Can you work these out from the model? Positions are in its coordinate system, mm. A direction names the side the tool comes from. Coordinates: 2 decimals unless noted, no trailing zeros. Write each loop counter-clockwise with the first axis right and the second up, starting at its lowest first coordinate (ties: lowest second). Pieces come first, ordered by that corner, then holes. Notation, with made-up numbers: (-18.75, 38) - (29.25, 38) arc R15 cw to (29.25, 51) - close; hole circle Ø10 at (72.5, 70). An arc over 180 degrees is marked (long way). Use one line per item in the form item = value. Start each with the question number.
(1) If we section it at D-D on y = -5: Please give me the cut outline in (x, z).
(2) On a 3-axis mill with a long thin cutter (end or side, diameter ignored), from which of +Z, -Z, +X, -X, +Y, -Y can I reach the whole of each face in a straight line? I mean faces 5 (the face through (51, 8, 1)), 6 (the face through (0.86, 15.1, 0.76)), 7 (the face through (41, -2, 2)), 8 (the face through (0.86, 0.9, 0.76)), 9 (the face through (10, -2, 2)). Say none if no direction works.
(3) If we section it at C-C on z = 2: Please give me the cut outline in (x, y).
(4) For pin 1 Ø0.8 at (x, z) = (15.5, 0.5) entering from +Y; pin 2 Ø0.8 at (x, z) = (46, 2.5) entering from -Y; pin 3 Ø1.5 at (y, z) = (-2.5, 0.5) entering from -X; pin 4 Ø1.2 at (y, z) = (-4, 2.5) entering from -X, each with a flat end and sliding along its axis, tell me the tip position at first contact or that it passes through.
(5) If I drill on probe 1 along X at (y, z) = (18, 2.25); probe 2 along X at (y, z) = (-5, 1.85); probe 3 along Y at (x, z) = (25.5, 1.9), over which ranges is the centre line in solid material (lowest first)? Write a range as from..to.
(6) If we section it at A-A on x = 25.5: Please give me the cut outline in (y, z).
(7) Thinking about a two-plate mould opening in Y: for faces 1 (the face through (-0.283, 17.024, 1.993)), 2 (the face through (23.6, 16.3, 1.5)), 3 (the face through (26, 20, 2)), 4 (the face through (51.04, 17.11, 1.99)), which applies, pulls with the +Y half, pulls with the -Y half, needs draft (parallel to the pull), parting line crosses it, or undercut?
(8) If we section it at B-B on y = 18: Please give me the cut outline in (x, z).
```python
from build123d import *

# Parameters (mm, degrees)
SKETCH_1_W                  = 51
SKETCH_1_H                  = 16
EXTRUDE_1_DEPTH             = 1.5
EXTRUDE_2_DEPTH             = 1.5
FILLET_2_R                  = 3
HOLE_WIZARD_M21_D           = 2
HOLE_WIZARD_M21_CSINK_D     = 3
HOLE_WIZARD_M21_CSINK_ANGLE = 90


with BuildPart() as part:
    # Эскиз1 → Бобышка-Вытянуть1 (new body)
    with BuildSketch(Plane.XY):
        with Locations((25.5, 8)):
            Rectangle(SKETCH_1_W, SKETCH_1_H)
    extrude(amount=EXTRUDE_1_DEPTH)

    # Эскиз2 → Бобышка-Вытянуть2 (add)
    with BuildSketch(Plane.XY.offset(1.5)):
        Polygon((3.5, 20), (47.5, 20), (53.5, 20), (53.5, 19.5), (53.5, -2), (28.75, -2), (28.75, -9), (21.75, -9), (21.75, -2), (-2.5, -2), (-2.5, 19.5), (-2.5, 20), align=None)
    extrude(amount=EXTRUDE_2_DEPTH)

    # Скругление2
    fillet_2_edges = [part.edges().sort_by_distance(p)[0] for p in [
        (0, 0, 0.75),
        (0, 16, 0.75),
        (51, 16, 0.75),
        (51, 0, 0.75),
    ]]
    fillet(fillet_2_edges, radius=FILLET_2_R)

    # Зенковка для  винта с полупотайной головкой M21 (through all)
    with Locations(Plane.XY.offset(3)):
        with Locations((25.5, -5), (-0.5, 18), (51.5, 18)):
            CounterSinkHole(HOLE_WIZARD_M21_D / 2, HOLE_WIZARD_M21_CSINK_D / 2, counter_sink_angle=HOLE_WIZARD_M21_CSINK_ANGLE)


solid = part.part
```
Reported:
q1.outline = (21.75, 1.5) - (24.5, 1.5) - (24.5, 2.5) - (24, 3) - (21.75, 3) - close; (26.5, 1.5) - (28.75, 1.5) - (28.75, 3) - (27, 3) - (26.5, 2.5) - close
q2.face_5 = -Z, +X, +Y, -Y
q2.face_6 = -Z, -X, +Y
q2.face_7 = +Z, -Z, +X, -Y
q2.face_8 = -Z, -X, -Y
q2.face_9 = +Z, -Z, -X, -Y
q3.outline = (-2.5, -2) - (21.75, -2) - (21.75, -9) - (28.75, -9) - (28.75, -2) - (53.5, -2) - (53.5, 20) - (-2.5, 20) - close; hole circle Ø2 at (-0.5, 18); hole circle Ø2 at (25.5, -5); hole circle Ø2 at (51.5, 18)
q4.pin_1 = 16
q4.pin_2 = -2
q4.pin_3 = through
q4.pin_4 = 21.75
q5.probe_1 = -2.5..-1.5, 0.5..50.5, 52.5..53.5
q5.probe_2 = 21.75..24.5, 26.5..28.75
q5.probe_3 = -9..-6, -4..20
q6.outline = (-9, 1.5) - (-6, 1.5) - (-6, 2.5) - (-6.5, 3) - (-9, 3) - close; (-4, 1.5) - (0, 1.5) - (0, 0) - (16, 0) - (16, 1.5) - (20, 1.5) - (20, 3) - (-3.5, 3) - (-4, 2.5) - close
q7.face_1 = undercut
q7.face_2 = needs draft
q7.face_3 = pulls with the +Y half
q7.face_4 = undercut
q8.outline = (-2.5, 1.5) - (-1.5, 1.5) - (-1.5, 2.5) - (-2, 3) - (-2.5, 3) - close; (0.5, 1.5) - (50.5, 1.5) - (50.5, 2.5) - (50, 3) - (1, 3) - (0.5, 2.5) - close; (52.5, 1.5) - (53.5, 1.5) - (53.5, 3) - (53, 3) - (52.5, 2.5) - close
